CAD build for the part. Positions are in the model's coordinates, mm. Round coordinates to 2 decimals unless told otherwise and drop trailing zeros. Order: outer loops, then holes, each group sorted by start corner. A loop starts at its lowest first (then second) coordinate and runs counter-clockwise, first axis right, second up. Notation, with made-up numbers: (36.25, -1) -> (51.25, -1) arc R20 cw to (51.25, 14) -> close; hole circle Ø4 at (-14.5, 77.5). An arc over 180 degrees is marked (long way). Return JSON: item names as keys, results as strings. Group by question number.
Q1. Cut at C-C (y = 0.2). Write the cut outline in (x, z).
Q2. Probe line 1 along X through (y, z) = (0.75, 0); line 2 along Z through (x, y) = (-24, 0.3); line 3 along Z through (x, y) = (27, 0.75). List the from-to ranges inside material, lowest first.
Q3. Cut at B-B (z = -1). Write the cut outline in (x, y), then the cut area to 3 significant figures.
from build123d import *

# Parameters (mm, degrees)
SKETCH_1_W          = 100
SKETCH_1_H          = 18
EXTRUDE_1_DEPTH     = 1
CHAMFER_1_SIZE      = 1
SKETCH_2_W          = 10
SKETCH_2_H          = 4
CUT_EXTRUDE_1_DEPTH = 1


with BuildPart() as part:
    # Эскиз1 → Бобышка-Вытянуть1 (new body)
    with BuildSketch(Plane(origin=(0, 0, 0), x_dir=(1, 0, 0), z_dir=(0, 1, 0))):
        Rectangle(SKETCH_1_W, SKETCH_1_H)
    extrude(amount=EXTRUDE_1_DEPTH)

    # Фаска1
    chamfer_1_edges = [part.edges().sort_by_distance(p)[0] for p in [
        (0, 1, 9),
    ]]
    chamfer(chamfer_1_edges, length=CHAMFER_1_SIZE - 0.0001)  # a hair under: the kernel refuses the full size

    # Эскиз2 → Вырез-Вытянуть1 (cut)
    with BuildSketch(Plane(origin=(0, 1, 0), x_dir=(1, 0, 0), z_dir=(0, 1, 0))):
        with Locations((-26, 0.5)):
            Rectangle(SKETCH_2_W, SKETCH_2_H)
        with Locations((26, 0.5)):
            Rectangle(SKETCH_2_W, SKETCH_2_H)
    extrude(amount=-CUT_EXTRUDE_1_DEPTH, mode=Mode.SUBTRACT)


solid = part.part
Solution:
{
 "1": {"outline": "(-50, -9) -> (50, -9) -> (50, 8.8) -> (-50, 8.8) -> close; hole (-31, -2.5) -> (-21, -2.5) -> (-21, 1.5) -> (-31, 1.5) -> close; hole (21, -2.5) -> (31, -2.5) -> (31, 1.5) -> (21, 1.5) -> close"},
 "2": {"line 1": "x = -50 to -31, -21 to 21, 31 to 50", "line 2": "z = -9 to -2.5, 1.5 to 8.7", "line 3": "z = -9 to -2.5, 1.5 to 8.25"},
 "3": {"outline": "(-50, 0) -> (-31, 0) -> (-31, 1) -> (-50, 1) -> close; (-21, 0) -> (21, 0) -> (21, 1) -> (-21, 1) -> close; (31, 0) -> (50, 0) -> (50, 1) -> (31, 1) -> close", "area": "80.0 mm²"}
}
